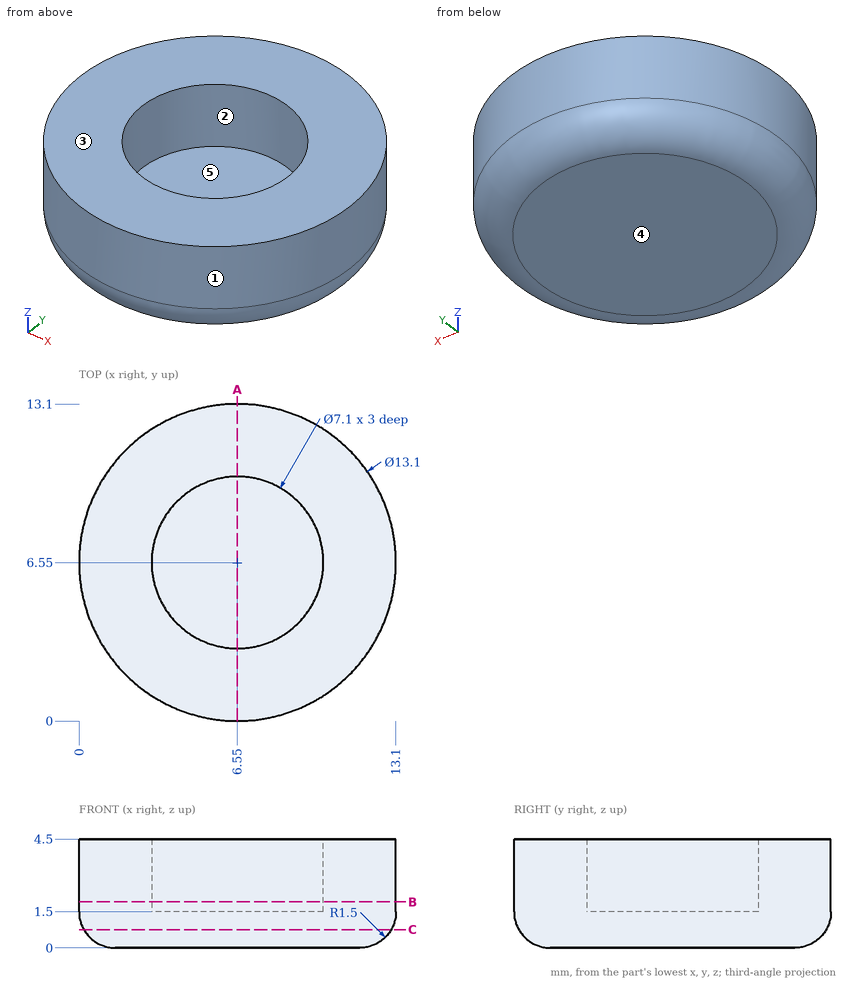
Input: dimensioned drawing with shaded views. Units: mm. Origin: part minimum x, y, z. A direction names the side the tool comes from. Coordinates: 2 decimals unless noted, no trailing zeros. Order: outer loops, then holes, each group sorted by start corner. A loop starts at its lowest first (then second) coordinate and runs counter-clockwise, first axis right, second up. Notation, with made-up numbers: (75.25, -11.5) - (92.25, -11.5) arc R18 cw to (92.25, 3.5) - close; hole circle Ø10 at (87, -12). An arc over 180 degrees is marked (long way). Put each result on its own line as item: value.
1. Contact query for flat-ended pins moving along their axis: pin 1 Ø2 at (x, z) = (8, 2) entering from +Y; pin 2 Ø1 at (x, y) = (6, 8.5) entering from +Z; pin 3 Ø1 at (y, z) = (11.5, 1.5) entering from +X. Output: stop coordinate, or through.
Report:
pin 1: stops at y = 13.08
pin 2: stops at z = 1.5
pin 3: stops at x = 11.36
2. Cut plane B-B on z = 1.9. Return the cut outline in (x, y), then the cut area to 3 significant figures.
Report:
outline: circle Ø13.1 at (6.55, 6.55); hole circle Ø7.1 at (6.55, 6.55)
area: 95.2 mm2
3. Draft query along Y for the marked faces 1, 2 and 3. Return one class per face: pulls with the +Y half, pulls with the -Y half, needs draft (parallel to the pull), parting line crosses it, or undercut.
Report:
face 1: parting line crosses it
face 2: undercut
face 3: needs draft
4. Cut plane C-C on z = 0.75. Return the cut outline in (x, y).
Report:
outline: circle Ø12.7 at (6.55, 6.55)
5. Cut plane A-A on x = 6.55. Return the cut outline in (y, z), then the cut area to 3 significant figures.
Report:
outline: (0, 1.5) arc R1.5 ccw to (1.5, 0) - (11.6, 0) arc R1.5 ccw to (13.1, 1.5) - (13.1, 4.5) - (10.1, 4.5) - (10.1, 1.5) - (3, 1.5) - (3, 4.5) - (0, 4.5) - close
area: 36.7 mm2
6. Line query: line 1 along Y through (x, z) = (6.55, 3.3); line 2 along Z through (x, y) = (4, 6); line 3 along X through (y, z) = (8.5, 1.8). Output: solid intervals per line, ascending.
Report:
line 1: y = 0 to 3, 10.1 to 13.1
line 2: z = 0 to 1.5
line 3: x = 0.3 to 3.58, 9.52 to 12.8
7. Reachability of the marked faces 4 and 5 from +Z, -Z, +X, -X, +Y, -Y: full face, straight path, thin tool, end or side. Return the list, or none.
Report:
face 4: -Z, +X, -X, +Y, -Y
face 5: +Z
